Work out the finished part from the listing and answer in its coordinate system (mm). A direction names the side the tool comes from. Give positions to 0.01 mm unless a question says otherwise; leave off trailing zeros. Order: outer loops, then holes, each group sorted by start corner. A loop starts at its lowest first (then second) coordinate and runs counter-clockwise, first axis right, second up. Notation, with made-up numbers: (72.5, -25.5) -> (77.5, -25.5) arc R27 ccw to (77.5, 11.5) -> close; hole circle Ø1 at (44.5, 19.25). An arc over 180 degrees is marked (long way). Answer as CSV lines item,"result". Start each with the question number.
1. A cutting plane is placed at C-C (z = 9.75). Give the vertices of the cut face in (x, y), then the cut area to 3 significant figures.
2. For faces 1 (the cylindrical face through (-25, 2.2, 2.6)), 2 (the flat face through (8, 4, 0)), 3 (the cylindrical face through (-7.026, 3.493, -0.391)), 4 (the flat face through (38, 4, 0)), 5 (the flat face through (-42, 4, 0)), determine the directions among +Z, -Z, +X, -X, +Y, -Y from which every point of the face is accessible in a straight line to the end or side of a thin tool.
3. Flat-ended cylindrical pins translate along their axes: pin 1 (0.8 mm diameter, centred on x = -27.5, z = 3.5, fed in from +Y); pin 2 (4 mm diameter, centred on x = 40, z = 0, fed in from +Y); pin 3 (2.5 mm diameter, centred on y = 7, z = 5.5, fed in from +X). Find the tip coordinate at first contact, or state that the pin passes through.
4. For a pull along X with two mould halves and no side action, classify faces 6 (the flat face through (-45, 1, 0)), 7 (the cylindrical face through (-11.66, 1.97, -0.37)), 8 (the flat face through (-1, 1, -4)) as released by +X, released by -X, zero draft, split by the parting line, or undercut.
5. A cutting plane is placed at D-D (z = 4.75). Give the vertices of the cut face in (x, y).
6. Find the intervals of material crossed by L1, parallel to X at y = 8.25, z = 8.75; L2, parallel to X at y = 1.55, z = 0; L3, parallel to Y at x = 25, z = 11.3, in increasing order.
7. A cutting plane is placed at A-A (x = 25). Give the vertices of the cut face in (y, z).
8. A cutting plane is placed at B-B (y = 5). Give the vertices of the cut face in (x, z).
from build123d import *

# Parameters (mm, degrees)
SKETCH_1_W          = 90
SKETCH_1_H          = 8
SKETCH_1_R          = 1.7
EXTRUDE_1_DEPTH     = 3
SKETCH_2_W          = 10
SKETCH_2_H          = 3
EXTRUDE_2_DEPTH     = 8
SKETCH_3_W          = 10
SKETCH_3_H          = 3
EXTRUDE_3_DEPTH     = 8
SKETCH_4_R          = 1.7
CUT_EXTRUDE_1_DEPTH = 49.114446895
EXTRUDE_4_DEPTH     = 2
EXTRUDE_5_DEPTH     = 2
SKETCH_7_R          = 2.8
CUT_EXTRUDE_2_DEPTH = 49.114446895
SKETCH_8_R          = 3
SKETCH_8_R_2        = 1.7
EXTRUDE_6_DEPTH     = 1


with BuildPart() as part:
    # 草图1 → 凸台-拉伸1 (new body)
    with BuildSketch(Plane(origin=(0, 0, 0), x_dir=(1, 0, 0), z_dir=(0, 1, 0))):
        Rectangle(SKETCH_1_W, SKETCH_1_H)
        with Locations(Location((-10, 0, 0), (0, 0, 270))):
            Circle(SKETCH_1_R, mode=Mode.SUBTRACT)
        with Locations(Location((10, 0, 0), (0, 0, 270))):
            Circle(SKETCH_1_R, mode=Mode.SUBTRACT)
        with Locations(Location((40, 0, 0), (0, 0, 270))):
            Circle(SKETCH_1_R, mode=Mode.SUBTRACT)
        with Locations(Location((-40, 0, 0), (0, 0, 270))):
            Circle(SKETCH_1_R, mode=Mode.SUBTRACT)
    extrude(amount=EXTRUDE_1_DEPTH)

    # 草图2 → 凸台-拉伸2 (add)
    with BuildSketch(Plane(origin=(0, 0, 4), x_dir=(-1, 0, 0), z_dir=(0, 0, -1))):
        with Locations((25, 1.5)):
            Rectangle(SKETCH_2_W, SKETCH_2_H)
    extrude_2 = extrude(amount=-EXTRUDE_2_DEPTH)

    # 草图3 → 凸台-拉伸3 (add)
    with BuildSketch(Plane(origin=(0, 3, 0), x_dir=(1, 0, 0), z_dir=(0, 1, 0))):
        with Locations((-25, -10.5)):
            Rectangle(SKETCH_3_W, SKETCH_3_H)
    extrude_3 = extrude(amount=EXTRUDE_3_DEPTH)

    # 草图4 → 切除-拉伸1 (cut, through all)
    with BuildSketch(Plane(origin=(0, 0, 9), x_dir=(-1, 0, 0), z_dir=(0, 0, -1))):
        with Locations((25, 5)):
            Circle(SKETCH_4_R)
    cut_extrude_1 = extrude(amount=-CUT_EXTRUDE_1_DEPTH, mode=Mode.SUBTRACT)

    # 草图5 → 凸台-拉伸4 (add)
    with BuildSketch(Plane(origin=(-20, 0, 0), x_dir=(0, 0, -1), z_dir=(1, 0, 0))):
        Polygon((-9, 11), (4, 3), (-9, 3), align=None)
    extrude_4 = extrude(amount=-EXTRUDE_4_DEPTH)

    # 草图6 → 凸台-拉伸5 (add)
    with BuildSketch(Plane.ZY.offset(30)):
        Polygon((9, 11), (-4, 3), (9, 3), align=None)
    extrude_5 = extrude(amount=-EXTRUDE_5_DEPTH)

    # 草图7 → 切除-拉伸2 (cut, through all)
    with BuildSketch(Plane(origin=(0, 0, 9), x_dir=(-1, 0, 0), z_dir=(0, 0, -1))):
        with Locations((25, 5)):
            Circle(SKETCH_7_R)
    cut_extrude_2 = extrude(amount=CUT_EXTRUDE_2_DEPTH, mode=Mode.SUBTRACT)

    # 镜向1: 凸台-拉伸2, 凸台-拉伸3, 切除-拉伸1, 凸台-拉伸4, 凸台-拉伸5, 切除-拉伸2 across plane
    add(extrude_2.mirror(Plane(origin=(0, 0, 0), x_dir=(0, 0, 1), z_dir=(1, 0, 0))))
    add(extrude_3.mirror(Plane(origin=(0, 0, 0), x_dir=(0, 0, 1), z_dir=(1, 0, 0))))
    add(cut_extrude_1.mirror(Plane(origin=(0, 0, 0), x_dir=(0, 0, 1), z_dir=(1, 0, 0))), mode=Mode.SUBTRACT)
    add(extrude_4.mirror(Plane(origin=(0, 0, 0), x_dir=(0, 0, 1), z_dir=(1, 0, 0))))
    add(extrude_5.mirror(Plane(origin=(0, 0, 0), x_dir=(0, 0, 1), z_dir=(1, 0, 0))))
    add(cut_extrude_2.mirror(Plane(origin=(0, 0, 0), x_dir=(0, 0, 1), z_dir=(1, 0, 0))), mode=Mode.SUBTRACT)

    # 草图8 → 凸台-拉伸6 (add)
    # profile 1 of 4: a face of its own
    with BuildSketch(Plane(origin=(0, 3, 0), x_dir=(1, 0, 0), z_dir=(0, 1, 0))):
        with Locations(Location((-40, 0, 0), (0, 0, 270))):
            Circle(SKETCH_8_R)
        with Locations(Location((-40, 0, 0), (0, 0, 270))):
            Circle(SKETCH_8_R_2, mode=Mode.SUBTRACT)
    # profile 2 of 4: a face of its own
    with BuildSketch(Plane(origin=(0, 3, 0), x_dir=(1, 0, 0), z_dir=(0, 1, 0))):
        with Locations(Location((-10, 0, 0), (0, 0, 270))):
            Circle(SKETCH_8_R)
        with Locations(Location((-10, 0, 0), (0, 0, 270))):
            Circle(SKETCH_8_R_2, mode=Mode.SUBTRACT)
    # profile 3 of 4: a face of its own
    with BuildSketch(Plane(origin=(0, 3, 0), x_dir=(1, 0, 0), z_dir=(0, 1, 0))):
        with Locations(Location((10, 0, 0), (0, 0, 270))):
            Circle(SKETCH_8_R)
        with Locations(Location((10, 0, 0), (0, 0, 270))):
            Circle(SKETCH_8_R_2, mode=Mode.SUBTRACT)
    # profile 4 of 4: a face of its own
    with BuildSketch(Plane(origin=(0, 3, 0), x_dir=(1, 0, 0), z_dir=(0, 1, 0))):
        with Locations(Location((40, 0, 0), (0, 0, 270))):
            Circle(SKETCH_8_R)
        with Locations(Location((40, 0, 0), (0, 0, 270))):
            Circle(SKETCH_8_R_2, mode=Mode.SUBTRACT)
    extrude(amount=EXTRUDE_6_DEPTH)


solid = part.part
Answer sheet:
1,outline,"(-30, 0) -> (-20, 0) -> (-20, 11) -> (-30, 11) -> close; (20, 0) -> (30, 0) -> (30, 11) -> (20, 11) -> close; hole circle Ø3.4 at (-25, 5); hole circle Ø3.4 at (25, 5)"
1,area,"202 mm^2"
2,face 1,"-Z, +Y"
2,face 2,"+Z, -Z, +Y"
2,face 3,"+Y"
2,face 4,"+Z, -Z, +X, +Y"
2,face 5,"+Z, -Z, -X, +Y"
3,pin 1,"stops at y = 3"
3,pin 2,"stops at y = 4"
3,pin 3,"stops at x = 30"
4,face 6,"released by -X"
4,face 7,"undercut"
4,face 8,"zero draft"
5,outline,"(-30, 0) -> (-20, 0) -> (-20, 8.38) -> (-22, 8.38) -> (-22, 3) -> (-23.04, 3) arc R2.8 cw to (-26.96, 3) -> (-28, 3) -> (-28, 8.38) -> (-30, 8.38) -> close; (20, 0) -> (30, 0) -> (30, 8.38) -> (28, 8.38) -> (28, 3) -> (26.96, 3) arc R2.8 cw to (23.04, 3) -> (22, 3) -> (22, 8.38) -> (20, 8.38) -> close"
6,L1,"x = -30 to -28, -22 to -20, 20 to 22, 28 to 30"
6,L2,"x = -45 to -41.7, -38.3 to -11.7, -8.3 to 8.3, 11.7 to 38.3, 41.7 to 45"
6,L3,"y = 0 to 3.3, 6.7 to 11"
7,outline,"(0, -4) -> (2.2, -4) -> (2.2, 9) -> (3.3, 9) -> (3.3, 12) -> (0, 12) -> close; (6.7, 9) -> (11, 9) -> (11, 12) -> (6.7, 12) -> close"
8,outline,"(-30, -0.75) -> (-28, -0.75) -> (-28, 9) -> (-26.7, 9) -> (-26.7, 12) -> (-30, 12) -> close; (-23.3, 9) -> (-22, 9) -> (-22, -0.75) -> (-20, -0.75) -> (-20, 12) -> (-23.3, 12) -> close; (20, -0.75) -> (22, -0.75) -> (22, 9) -> (23.3, 9) -> (23.3, 12) -> (20, 12) -> close; (26.7, 9) -> (28, 9) -> (28, -0.75) -> (30, -0.75) -> (30, 12) -> (26.7, 12) -> close"
